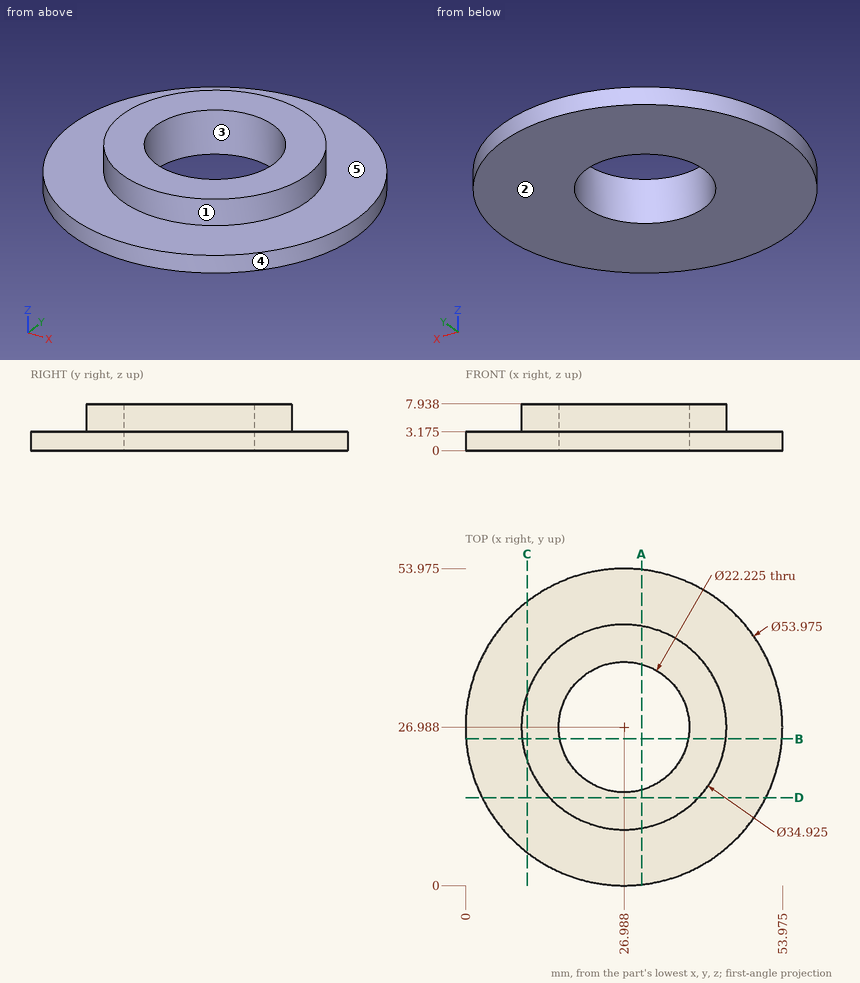
Print and shaded views of the part. All mm, measured from the part's lowest x, y and z. A direction names the side the tool comes from. Coordinates: 2 decimals unless noted, no trailing zeros. Order: outer loops, then holes, each group sorted by start corner. A loop starts at its lowest first (then second) coordinate and runs counter-clockwise, first axis right, second up. Notation, with made-up numbers: (79.25, 85) - (100.25, 85) arc R21 ccw to (100.25, 93) - close; hole circle Ø1 at (54, 57.5). An arc over 180 degrees is marked (long way). Return JSON: item names as keys, results as strings. Group by question number.
Item 1: Cut at A-A (x = 30). List the corners of the cut face in (y, z) (1 decimal), plus the area to 3 significant figures.
Item 2: Drill centre lines: probe 1 along Z at (x, y) = (42, 17.5) (1 decimal); probe 2 along Y at (x, z) = (33, 0.5) (1 decimal); probe 3 along Y at (x, z) = (20, 5.5) (1 decimal). Where is each one in solid material? Low to high. Write a range as from..to.
Item 3: Pull direction X, two halves, no side cores. Call the marked faces 1, 2 and 3: pulls with the +X half, pulls with the -X half, needs draft (parallel to the pull), parting line crosses it, or undercut.
Item 4: Which spindle directions (+Z, -Z, +X, -X, +Y, -Y) get a long thin tool onto all of the face, cutting with end or side? Do the marked faces 4 and 5. Say none if no direction does.
Item 5: Cut at D-D (y = 15). List the corners of the cut face in (x, z) (1 decimal).
Item 6: Cut at C-C (x = 10.5). List the corners of the cut face in (y, z) (1 decimal).
Item 7: Cut at B-B (y = 25). List the corners of the cut face in (x, z) (1 decimal).
Item 8: Pin check, flat tips, straight feed: pin 1 (2 mm diameter, centred on y = 8.5, z = 3.5, fed in from -X); pin 2 (1 mm diameter, centred on x = 12.5, y = 40.5, fed in from +Z) (1 decimal); pin 3 (3 mm diameter, centred on x = 15, z = 6, fed in from -Y) (1 decimal). Stop position of each tip, or through.
Check values:
{
 "1": {"outline": "(0.2, 0) - (16.3, 0) - (16.3, 7.9) - (9.8, 7.9) - (9.8, 3.2) - (0.2, 3.2) - close; (37.7, 0) - (53.8, 0) - (53.8, 3.2) - (44.2, 3.2) - (44.2, 7.9) - (37.7, 7.9) - close", "area": "164 mm2"},
 "2": {"probe 1": "z = 0..3.2", "probe 2": "y = 0.7..17.6, 36.3..53.3", "probe 3": "y = 11..18.3, 35.6..43"},
 "3": {"face 1": "parting line crosses it", "face 2": "needs draft", "face 3": "undercut"},
 "4": {"face 4": "+Z, -Z", "face 5": "+Z"},
 "5": {"outline": "(2.8, 0) - (51.2, 0) - (51.2, 3.2) - (39.7, 3.2) - (39.7, 7.9) - (14.3, 7.9) - (14.3, 3.2) - (2.8, 3.2) - close"},
 "6": {"outline": "(5.6, 0) - (48.4, 0) - (48.4, 3.2) - (32.7, 3.2) - (32.7, 7.9) - (21.2, 7.9) - (21.2, 3.2) - (5.6, 3.2) - close"},
 "7": {"outline": "(0.1, 0) - (16.1, 0) - (16.1, 7.9) - (9.6, 7.9) - (9.6, 3.2) - (0.1, 3.2) - close; (37.9, 0) - (53.9, 0) - (53.9, 3.2) - (44.3, 3.2) - (44.3, 7.9) - (37.9, 7.9) - close"},
 "8": {"pin 1": "stops at x = 6.48", "pin 2": "stops at z = 3.2", "pin 3": "stops at y = 13"}
}
